CAD build for the part. Positions are in the model's coordinates, mm. A direction names the side the tool comes from. Round coordinates to 2 decimals unless told otherwise and drop trailing zeros. Order: outer loops, then holes, each group sorted by start corner. A loop starts at its lowest first (then second) coordinate and runs counter-clockwise, first axis right, second up. Notation, with made-up numbers: M 85.25,75 L 104.25,75 A34 cw 104.25,110 Z; hole C 17,-36 d2. An arc over 180 degrees is marked long. Answer as a JSON object with one key per item and string values.
Autodesk Inventor part; units mm, degrees
ref_plane "YZ Plane" through (0, 0, 0) normal (1, 0, 0) x (0, 1, 0)
ref_plane "XZ Plane" through (0, 0, 0) normal (0, 1, 0) x (-1, 0, 0)
ref_plane "XY Plane" through (0, 0, 0) normal (0, 0, 1) x (1, 0, 0)
sketch "Esboço1" plane through (0, 0, 0) normal (1, 0, 0) x (0, 1, 0)
  line L0 (40.5, 60) -> (-42.5, 60)
  line L1 (-42.5, 60) -> (-42.5, -60)
  line L2 (-42.5, -60) -> (40.5, -60)
  line L3 (42.5, -58) -> (42.5, 58)
  line L4 (-42.5, 60) -> (42.5, -60) construction
  arc A0 (42.5, 58) -> (40.5, 60) centre (40.5, 58) ccw
  arc A1 (40.5, -60) -> (42.5, -58) centre (40.5, -58) ccw
  point P0 (0, 0)
  dimension "d0" = 85
  dimension "d1" = 120
  dimension "d4" = 2
extrude "Extrusão1" add sketch "Esboço1" along normal blind 5
sketch "Esboço2" plane through (5, 0, 0) normal (1, 0, 0) x (0, 0, -1)
  line L0 (-60, 40.5) -> (-60, -42.5)
  line L1 (-60, -42.5) -> (-58.5, -42.5)
  line L2 (-60, -42.5) -> (60, -42.5)
  line L3 (60, -42.5) -> (58.5, -42.5)
  arc A0 (-58, 42.5) -> (-60, 40.5) centre (-58, 40.5) ccw
  line L4 (-58, 42.5) -> (-58, 41)
  line L5 (-58.5, -42.5) -> (-56.5, -42.5)
  line L6 (-56.5, -42.5) -> (-56.5, 37)
  line L7 (-56.5, 41) -> (-56.5, 41)
  line L8 (-58.5, 39) -> (-58.5, -42.5)
  line L9 (58.5, -42.5) -> (56.5, -42.5)
  line L10 (56.5, -42.5) -> (56.5, 37)
  line L11 (56.5, 41) -> (56.5, 41)
  line L12 (58.5, 39) -> (58.5, -42.5)
  line L13 (-56.5, 41) -> (56.5, 41)
  line L14 (54.5, 39) -> (-54.5, 39)
  arc A1 (-56.5, 41) -> (-58.5, 39) centre (-56.5, 39) ccw
  arc A2 (-54.5, 39) -> (-56.5, 37) centre (-54.5, 37) ccw
  arc A3 (58.5, 39) -> (56.5, 41) centre (56.5, 39) ccw
  arc A4 (56.5, 37) -> (54.5, 39) centre (54.5, 37) ccw
  point P0 (0, 0)
  point P1 (-58.5, 41)
  point P2 (58.5, 41)
  dimension "d7" = 1.5
  dimension "d8" = 1.5
  dimension "d9" = 1.5
  dimension "d10" = 2
  dimension "d11" = 2
  dimension "d13" = 2
extrude "Extrusão2" add sketch "Esboço2" along normal blind 6 contours L8 A1 L13 A3 L12 L2 L10 A4 L14 A2 L6
sketch "Esboço3" plane through (11, 0, 0) normal (1, 0, 0) x (0, 0, -1)
  circle A0 centre (-57, 39.5) radius 1.6
  circle A1 centre (57, 39.5) radius 1.6
  point P0 (0, 0)
  dimension "d18" = 3.2
hole "Furo1" at (11, 39.5, 57) direction (-1, 0, 0) diameter 3.302 depth 40 tip angle 118
hole "Furo2" at (11, 39.5, -57) direction (-1, 0, 0) diameter 3.302 depth 40 tip angle 118
sketch "Esboço4" plane through (5, 0, 0) normal (1, 0, 0) x (0, 0, -1)
  line L0 (-60, -42.5) -> (60, -42.5)
  line L1 (-60, -42.5) -> (60, -42.5)
  line L2 (60, -42.5) -> (60, -47.5)
  line L3 (60, -47.5) -> (-60, -47.5)
  line L4 (-60, -47.5) -> (-60, -42.5)
  point P0 (0, 0)
  point P1 (60, -42.5)
  dimension "d33" = 5
extrude "Extrusão3" add sketch "Esboço4" against normal blind 5
sketch "Esboço5" plane through (5, 0, 0) normal (1, 0, 0) x (0, 0, -1)
  line L0 (-60, 40.5) -> (-60, -47.5)
  line L1 (60, 40.5) -> (60, -47.5)
  line L2 (-60, -47.5) -> (60, -47.5)
  line L3 (60, -47.5) -> (60, -42.5)
  line L4 (60, -42.5) -> (-60, -42.5)
  line L5 (-60, -42.5) -> (-60, -47.5)
  point P0 (0, 0)
  point P1 (60, -47.5)
  dimension "d36" = 5
extrude "Extrusão4" add sketch "Esboço5" along normal blind 53.158
sketch "Esboço6" plane through (11, 0, 0) normal (1, 0, 0) x (0, 0, -1)
  line L0 (60, -42.5) -> (-60, -42.5)
  line L1 (-58.4844, -42.5) -> (-56.4844, -42.5)
  line L2 (-56.4844, -42.5) -> (-56.4844, -39.5)
  line L3 (-56.4844, -39.5) -> (-58.4844, -39.5)
  line L4 (-58.4844, -39.5) -> (-58.4844, -42.5)
  line L5 (56.5, 37) -> (56.5, -42.5)
  line L6 (58.5, 38.8102) -> (58.5, -42.5)
  line L7 (56.5, -42.5) -> (58.5, -42.5)
  line L8 (58.5, -42.5) -> (58.5, -39.5)
  line L9 (58.5, -39.5) -> (56.5, -39.5)
  line L10 (56.5, -39.5) -> (56.5, -42.5)
  point P0 (0, 0)
  dimension "d39" = 2
  dimension "d40" = 3
  dimension "d41" = 3
extrude "Extrusão5" add sketch "Esboço6" along normal blind 47.158
chamfer "Chanfro1" distance 2 angle 45 2 edges at (58.158, -39.5, 57.4844) (58.158, -39.5, -57.5)
chamfer "Chanfro2" distance 4 angle 45 1 edges at (0, -47.5, 0)
chamfer "Chanfro3" distance 2 angle 45 1 edges at (58.158, -47.5, 0)
sketch "Esboço7" plane through (5, 0, 0) normal (1, 0, 0) x (0, 0, -1)
  circle A0 centre (-45, 0) radius 3
  circle A1 centre (45, 0) radius 3
  point P0 (0, 0)
  dimension "d61" = 6
  dimension "d62" = 6
hole "Furo3" at (5, 0, 45) direction (-1, 0, 0) diameter 6.4008 depth 22.931 tip angle 118
hole "Furo4" at (5, 0, -45) direction (-1, 0, 0) diameter 6.4008 depth 22.931 tip angle 118
sketch "Esboço8" plane through (5, -42.5, 56.5) normal (0, 1, 0) x (1, 0, 0)
  line L0 (0, 0) -> (0, 113)
  line L1 (0, 0) -> (30, 0)
  line L2 (0, 56.5) -> (0, 0)
  line L3 (22.5, 47) -> (37.5, 47)
  line L4 (39.5, 49) -> (39.5, 64)
  line L5 (37.5, 66) -> (22.5, 66)
  line L6 (20.5, 64) -> (20.5, 49)
  line L7 (20.5, 47) -> (39.5, 66) construction
  line L8 (39.5, 47) -> (20.5, 66) construction
  line L9 (22.5, 12) -> (37.5, 12)
  line L10 (39.5, 14) -> (39.5, 29)
  line L11 (37.5, 31) -> (22.5, 31)
  line L12 (20.5, 29) -> (20.5, 14)
  line L13 (20.5, 12) -> (39.5, 31) construction
  line L14 (39.5, 12) -> (20.5, 31) construction
  line L15 (22.5, 82) -> (37.5, 82)
  line L16 (39.5, 84) -> (39.5, 99)
  line L17 (37.5, 101) -> (22.5, 101)
  line L18 (20.5, 99) -> (20.5, 84)
  line L19 (20.5, 82) -> (39.5, 101) construction
  line L20 (39.5, 82) -> (20.5, 101) construction
  arc A0 (20.5, 14) -> (22.5, 12) centre (22.5, 14) ccw
  arc A1 (22.5, 31) -> (20.5, 29) centre (22.5, 29) ccw
  arc A2 (39.5, 29) -> (37.5, 31) centre (37.5, 29) ccw
  arc A3 (37.5, 12) -> (39.5, 14) centre (37.5, 14) ccw
  arc A4 (37.5, 47) -> (39.5, 49) centre (37.5, 49) ccw
  arc A5 (39.5, 64) -> (37.5, 66) centre (37.5, 64) ccw
  arc A6 (22.5, 66) -> (20.5, 64) centre (22.5, 64) ccw
  arc A7 (20.5, 49) -> (22.5, 47) centre (22.5, 49) ccw
  arc A8 (22.5, 101) -> (20.5, 99) centre (22.5, 99) ccw
  arc A9 (39.5, 99) -> (37.5, 101) centre (37.5, 99) ccw
  arc A10 (20.5, 84) -> (22.5, 82) centre (22.5, 84) ccw
  arc A11 (37.5, 82) -> (39.5, 84) centre (37.5, 84) ccw
  point P0 (-5, 56.5)
  dimension "d82" = 19
  dimension "d83" = 19
  dimension "d88" = 19
  dimension "d89" = 19
  dimension "d91" = 19
  dimension "d92" = 19
  dimension "d93" = 2
  dimension "d94" = 2
extrude "Extrusão6" cut sketch "Esboço8" against normal through all
properties part number "sUPORTE"
Item 1: Wall check: line 1 along Z through (x, y) = (3, 0); line 2 along Y through (x, z) = (4, -57); line 3 along Y through (x, z) = (1, -45). Give the ranges that are in metal, low to high. Write a range as [from, to].
Worked answers:
{"line 1": "z = [-60, -48.2], [-41.8, 41.8], [48.2, 60]", "line 2": "y = [-47.5, 37.85], [41.15, 42.5]", "line 3": "y = [-44.5, -3.2], [3.2, 42.5]"}
Item 2: 3-axis set-ups, long thin cutter, end or side, ignore diameter. For faces 4 (the flat face through (25, -42.5, -1)), 5 (the flat face through (34, -41, 56.484)), 6 (the flat face through (34, -41, 58.484)), 7 (the flat face through (44.5, -45, 0)): which of +Z, -Z, +X, -X, +Y, -Y reach the whole face in a straight line?
Worked answers:
{"face 4": "+X", "face 5": "+X, +Y", "face 6": "+Z, +X, +Y", "face 7": "+Y, -Y"}
Item 3: Saw through at A-A on y = 0. List the corners of the cut face in (x, z).
Worked answers:
{"outline": "M 0,-60 L 5,-60 L 5,-58.5 L 11,-58.5 L 11,-56.5 L 5,-56.5 L 5,-48.2 L 0,-48.2 Z; M 0,-41.8 L 5,-41.8 L 5,41.8 L 0,41.8 Z; M 0,48.2 L 5,48.2 L 5,56.5 L 11,56.5 L 11,58.5 L 5,58.5 L 5,60 L 0,60 Z"}
Item 4: Two-plate mould, pull along Z, no slides. Class faces 1 (the flat face through (2, 42.5, -1)), 2 (the flat face through (3, -16, 60)), 3 (the flat face through (5, -1, 1)): released by +Z, released by -Z, zero draft, split by the parting line, or undercut.
Worked answers:
{"face 1": "zero draft", "face 2": "released by +Z", "face 3": "undercut"}
Item 5: Saw through at B-B on z = -39. List the corners of the cut face in (x, y).
Worked answers:
{"outline": "M 0,-43.5 L 4,-47.5 L 25.5,-47.5 L 25.5,-42.5 L 5,-42.5 L 5,39 L 11,39 L 11,41 L 5,41 L 5,42.5 L 0,42.5 Z; M 44.5,-47.5 L 56.16,-47.5 L 58.16,-45.5 L 58.16,-42.5 L 44.5,-42.5 Z"}
Item 6: Drop flat-ended pins along their axis: pin 1 Ø5 at (y, z) = (11, -38) entering from +X; pin 2 Ø2 at (y, z) = (39.5, 57) entering from -X (1 decimal); pin 3 Ø2 at (x, z) = (42, -57) entering from +Y; pin 4 Ø12 at (x, z) = (45, -38.5) entering from +Y. Give the stop position or say it passes through.
Worked answers:
{"pin 1": "stops at x = 5", "pin 2": "passes through", "pin 3": "stops at y = -39.5", "pin 4": "stops at y = -42.5"}
